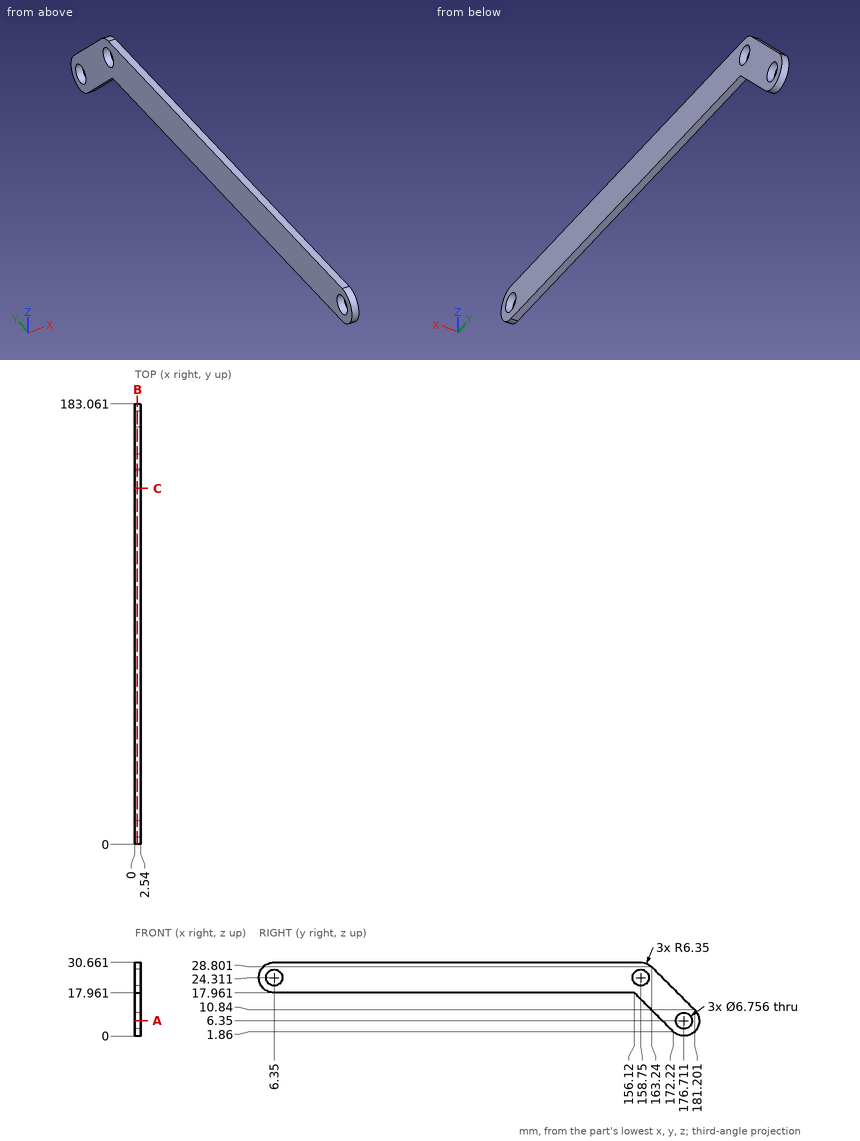
The figure shows three views and two pictorial views of one solid part (mm, origin at its lowest corner). Answer the questions. Coordinates: 2 decimals unless noted, no trailing zeros. Loops run counter-clockwise (first coordinate to the right, second up) from the corner with the lowest first, then second, coordinate; pieces in that order, holes last.
1) Find section B-B on x = 1.05. Write down the section's boundary in (y, z).
2) Flat-ended cylindrical pins translate along their axes: pin 1 Ø4 at (y, z) = (176.71, 6.35) entering from -X; pin 2 Ø8 at (y, z) = (157, 21) entering from -X. Find the tip coordinate at first contact, or state that the pin passes through.
3) Find the intervals of material crossed by L1, parallel to Z at x = 0.9, y = 6.35; L2, parallel to Z at x = 2.1, y = 40; L3, parallel to Y at x = 0.9, z = 24 (1 decimal), in increasing order.
4) Find section C-C on y = 148. Write down the section's boundary in (x, z).
5) Find section A-A on z = 6.35. Write down the section's boundary in (x, y), then the cut area to 3 significant figures.
Values:
1. outline: (6.35, 17.96) - (156.12, 17.96) - (172.22, 1.86) arc R6.35 ccw to (181.2, 10.84) - (163.24, 28.8) arc R6.35 ccw to (158.75, 30.66) - (6.35, 30.66) arc R6.35 ccw to start; hole circle Ø6.76 at (6.35, 24.31); hole circle Ø6.76 at (158.75, 24.31); hole circle Ø6.76 at (176.71, 6.35)
2. pin 1: passes through
2. pin 2: stops at x = 0
3. L1: z = 17.96 to 20.93, 27.69 to 30.66
3. L2: z = 17.96 to 30.66
3. L3: y = 0 to 3, 9.7 to 155.4, 162.1 to 168
4. outline: (0, 17.96) - (2.54, 17.96) - (2.54, 30.66) - (0, 30.66) - close
5. outline: (0, 167.73) - (2.54, 167.73) - (2.54, 173.33) - (0, 173.33) - close; (0, 180.09) - (2.54, 180.09) - (2.54, 183.06) - (0, 183.06) - close
5. area: 21.8 mm2
